Read the model definition and answer for the solid it produces. Units are mm, in the model's axes. A direction names the side the tool comes from. Round coordinates to 2 decimals unless told otherwise and drop trailing zeros. Loops run counter-clockwise (first coordinate to the right, second up) from the corner with the lowest first, then second, coordinate; pieces in that order, holes last. Notation, with made-up numbers: (-19, 59) - (-15, 59) arc R24 ccw to (-15, 76) - close; hole circle Ø8 at (-27, 11.5). An arc over 180 degrees is marked (long way). Answer as CSV lines item,"result".
Autodesk Inventor part; units mm, degrees
ref_plane "YZ Plane" through (0, 0, 0) normal (1, 0, 0) x (0, 1, 0)
ref_plane "XZ Plane" through (0, 0, 0) normal (0, 1, 0) x (-1, 0, 0)
ref_plane "XY Plane" through (0, 0, 0) normal (0, 0, 1) x (1, 0, 0)
sketch "Sketch1" plane through (0, 0, 0) normal (0, 0, 1) x (1, 0, 0)
  circle A0 centre (0, 0) radius 6
  line L0 (0, -35) -> (0, 80) construction
  line L1 (4, -35) -> (4, 80)
  line L2 (-4, 80) -> (-4, -35)
  arc A1 (-4, -35) -> (4, -35) centre (0, -35) ccw
  arc A2 (4, 80) -> (-4, 80) centre (0, 80) ccw
  point P0 (0, 22.5)
  dimension "d0" = 12
  dimension "d1" = 8
  dimension "d2" = 80
  dimension "d12" = 35
extrude "Extrusion1" add sketch "Sketch1" along normal mid plane 2.8
sketch "Sketch2" plane through (0, 0, 1.4) normal (0, 0, 1) x (1, 0, 0)
  arc A0 (4, 80) -> (-4, 80) centre (0, 80) ccw construction
  arc A1 (-4, 4.4721) -> (4, 4.4721) centre (0, 0) ccw construction
  circle A2 centre (0, 0) radius 1.75
  circle A3 centre (0, 80) radius 1.75
  line L0 (0, 12.7) -> (0, 5.7) construction
  line L1 (-1.3, 11.4) -> (-1.3, 7)
  line L2 (1.3, 7) -> (1.3, 11.4)
  arc A4 (1.3, 11.4) -> (-1.3, 11.4) centre (0, 11.4) ccw
  arc A5 (-1.3, 7) -> (1.3, 7) centre (0, 7) ccw
  arc A6 (-4, -35) -> (4, -35) centre (0, -35) ccw construction
  circle A7 centre (0, -35) radius 1.75
  point P0 (0, 9.2)
  dimension "d5" = 7
  dimension "d6" = 2.6
  dimension "d7" = 7
  dimension "d8" = 3.5
  dimension "d9" = 3.5
  dimension "d13" = 3.5
extrude "Extrusion2" cut sketch "Sketch2" against normal blind 3.5 contours A2 | A3 | A7
equation "\"d10\" = d13"
1) Find the intervals of material crossed by line 1 (Y direction, x = 0, z = -0.4); line 2 (X direction, y = 80, z = -0.45); line 3 (Y direction, x = -1, z = 0.6), in increasing order.
Entries:
line 1,"y = -39 to -36.75, -33.25 to -1.75, 1.75 to 78.25, 81.75 to 84"
line 2,"x = -4 to -1.75, 1.75 to 4"
line 3,"y = -38.87 to -36.44, -33.56 to -1.44, 1.44 to 78.56, 81.44 to 83.87"
2) The mould has two halves that part along Y. Classify faces 5 (the face through (1.669, -34.474, 0.02)), 6 (the face through (0, 23, 1.4)), 7 (the face through (0, -39, 0)): pulls with the +Y half, pulls with the -Y half, needs draft (parallel to the pull), parting line crosses it, or undercut.
Entries:
face 5,"undercut"
face 6,"needs draft"
face 7,"pulls with the -Y half"
3) A cutting plane is placed at C-C, the plane y = 28. Determine the outline of the cut face in (x, z).
Entries:
outline,"(-4, -1.4) - (4, -1.4) - (4, 1.4) - (-4, 1.4) - close"
4) A cutting plane is placed at B-B, the plane z = 0.9. Determine the outline of the cut face in (x, y).
Entries:
outline,"(-4, -35) arc R4 ccw to (4, -35) - (4, -4.47) arc R6 ccw to (4, 4.47) - (4, 80) arc R4 ccw to (-4, 80) - (-4, 4.47) arc R6 ccw to (-4, -4.47) - close; hole circle Ø3.5 at (0, -35); hole circle Ø3.5 at (0, 0); hole circle Ø3.5 at (0, 80)"
5) A cutting plane is placed at A-A, the plane y = 0. Determine the outline of the cut face in (x, z).
Entries:
outline,"(-6, -1.4) - (-1.75, -1.4) - (-1.75, 1.4) - (-6, 1.4) - close; (1.75, -1.4) - (6, -1.4) - (6, 1.4) - (1.75, 1.4) - close"
6) Each of these flat-tipped pins is pushed along its axis until it touches: P1, Ø1, axis at x = 2, z = 0, coming from the -Y side; P2, Ø3, axis at x = 0, y = 0, coming from the +Z side; P3, Ø1.4, axis at y = -18.5, z = 0, coming from the -X side; P4, Ø5.5, axis at x = 0, y = -35, coming from the -Z side. Where does it stop, or does it pass through?
Entries:
P1,"stops at y = -38.71"
P2,"passes through"
P3,"stops at x = -4"
P4,"stops at z = -1.4"
7) A cutting plane is placed at D-D, the plane x = 2.75. Determine the outline of the cut face in (y, z), plus the area to 3 significant figures.
Entries:
outline,"(-37.9, -1.4) - (82.9, -1.4) - (82.9, 1.4) - (-37.9, 1.4) - close"
area,"338 mm^2"
8) A tool of negligible diameter and unlimited length cuts with its end or side. For faces 1 (the face through (-4, -20, 0)), 2 (the face through (-4, 43, 0)), 3 (the face through (4, 42, 0)), 4 (the face through (4, -20, 0)), from which of +Z, -Z, +X, -X, +Y, -Y can it reach the whole face along a straight path? Write none if from no direction.
Entries:
face 1,"+Z, -Z, -X, -Y"
face 2,"+Z, -Z, -X, +Y"
face 3,"+Z, -Z, +X, +Y"
face 4,"+Z, -Z, +X, -Y"
